```python
from build123d import *

# Parameters (mm, degrees)
SKETCH1_W                 = 131.85
SKETCH1_H                 = 70
BOSS_EXTRUDE1_DEPTH       = 1.5
CUT_EXTRUDE1_REACH        = 137.268
SKETCH4_W                 = 8
SKETCH4_H                 = 4.5
SKETCH4_W_2               = 5
SKETCH4_H_2               = 1.5
BOSS_EXTRUDE2_DEPTH       = 3
MIRROR2_COPY_1_SKETCH_W   = 8
MIRROR2_COPY_1_SKETCH_H   = 4.5
MIRROR2_COPY_1_SKETCH_W_2 = 5
MIRROR2_COPY_1_SKETCH_H_2 = 1.5
MIRROR2_COPY_1_DEPTH      = 3
CUT_EXTRUDE2_REACH        = 137.335
CUT_EXTRUDE3_DEPTH        = 0.5


with BuildPart() as part:
    # Sketch1 → Boss-Extrude1 (new body)
    with BuildSketch(Plane.XY):
        with Locations((55.175, 25.25)):
            Rectangle(SKETCH1_W, SKETCH1_H)
    extrude(amount=BOSS_EXTRUDE1_DEPTH)

    # Sketch2 → Cut-Extrude1 (cut, up to next)
    with BuildSketch(Plane.XY.offset(1.5), mode=Mode.PRIVATE) as cut_extrude1_sk1:
        with BuildLine():
            Line((92.957060126, 22.2), (92.9875, 22.2))
            ThreePointArc((92.9875, 22.2), (96.0375, 25.25), (92.9875, 28.3))
            Line((92.9875, 28.3), (92.957060126, 28.3))
            ThreePointArc((92.957060126, 28.3), (81.0375, 25.25), (92.957060126, 22.2))
        make_face()
    cut_extrude1_tool1 = extrude(cut_extrude1_sk1.sketch, amount=-CUT_EXTRUDE1_REACH, mode=Mode.PRIVATE) & part.part
    add(cut_extrude1_tool1.solids().sort_by_distance((87.98685, 25.25, 1.5))[0], mode=Mode.SUBTRACT)

    # Sketch4 → Boss-Extrude2 (add)
    with BuildSketch(Plane(origin=(0, 0, 0), x_dir=(-1, 0, 0), z_dir=(0, 0, -1))):
        with Locations((-115.6, 56.5)):
            Rectangle(SKETCH4_W, SKETCH4_H)
        with Locations((-115.6, 56.5)):
            Rectangle(SKETCH4_W_2, SKETCH4_H_2, mode=Mode.SUBTRACT)
    boss_extrude2 = extrude(amount=BOSS_EXTRUDE2_DEPTH)

    # Mirror1: Boss-Extrude2 across plane
    add(boss_extrude2.mirror(Plane.ZX.offset(25.25)))

    # Mirror2: Boss-Extrude2 across plane
    add(boss_extrude2.mirror(Plane(origin=(55.175, 0, 0), x_dir=(0, 0, 1), z_dir=(1, 0, 0))))

    # Mirror2 copy 1 sketch → Mirror2 copy 1 (add)
    with BuildSketch(Plane(origin=(110.35, 50.5, 0), x_dir=(1, 0, 0), z_dir=(0, 0, -1))):
        with Locations((-115.6, 56.5)):
            Rectangle(MIRROR2_COPY_1_SKETCH_W, MIRROR2_COPY_1_SKETCH_H)
        with Locations((-115.6, 56.5)):
            Rectangle(MIRROR2_COPY_1_SKETCH_W_2, MIRROR2_COPY_1_SKETCH_H_2, mode=Mode.SUBTRACT)
    extrude(amount=MIRROR2_COPY_1_DEPTH)

    # Sketch5 → Cut-Extrude2 (cut, up to next)
    with BuildSketch(Plane.XY.offset(1.5), mode=Mode.PRIVATE) as cut_extrude2_sk1:
        with BuildLine():
            Line((90.774215328, 6.046350365), (96.908092333, 0.244034279))
            ThreePointArc((96.908092333, 0.244034279), (60.630444856, 25.25), (96.908092333, 50.255965721))
            Line((96.908092333, 50.255965721), (90.774215328, 44.453649635))
            ThreePointArc((90.774215328, 44.453649635), (67.8875, 25.25), (90.774215328, 6.046350365))
        make_face()
    cut_extrude2_tool1 = extrude(cut_extrude2_sk1.sketch, amount=-CUT_EXTRUDE2_REACH, mode=Mode.PRIVATE) & part.part
    add(cut_extrude2_tool1.solids().sort_by_distance((61.276961, 25.25, 1.5))[0], mode=Mode.SUBTRACT)

    # Sketch6 → Cut-Extrude3 (cut)
    with BuildSketch(Plane.XY.offset(1.5)):
        Polygon((-5.119922612, 25.25), (43.3775, -2.75), (43.3775, 6.583333333), (11.045884925, 25.25), (43.3775, 43.916666667), (43.3775, 53.25), align=None)
    extrude(amount=-CUT_EXTRUDE3_DEPTH, mode=Mode.SUBTRACT)


solid = part.part
```
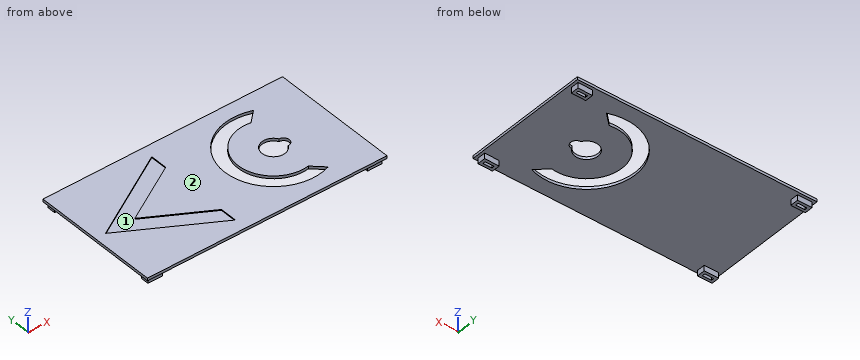
Geometry: final body of the model. Coordinates: model frame, mm. Face numbers are marked on the shaded views. Coordinates: 2 decimals unless noted, no trailing zeros. Order: outer loops, then holes, each group sorted by start corner. A loop starts at its lowest first (then second) coordinate and runs counter-clockwise, first axis right, second up. Notation, with made-up numbers: (69, 64) -> (117, 64) arc R14 ccw to (117, 79) -> close; hole circle Ø11 at (-33.75, 58). An arc over 180 degrees is marked (long way). Write each question's results on one line, items separated by ' | '. Start each with the question number.
1) Material intervals for line 1 along X through (y, z) = (25.25, 0.7); line 2 along X through (y, z) = (56, -0.45); line 3 along Y through (x, z) = (29, 1.25), sorted ascending.
2) First-contact query: pin 1 (2.5 mm diameter, centred on y = 56.5, z = -1.5, fed in from -X); pin 2 (0.9 mm diameter, centred on x = 115.5, z = -2, fed in from -Y); pin 3 (1 mm diameter, centred on x = 45, y = 22, fed in from -Z); pin 4 (2.5 mm diameter, centred on y = -6.5, z = -1, fed in from -X). Flat tips, straight axial feed; report the tip coordinate or a pass-through.
3) Cut plane C-C, the plane x = 105.5. Output: boundary loops of the cut face in (y, z), and give its area (3 significant figures).
4) Cut plane A-A, the plane z = -1.4. State how many separate pieces and enclosed holes the cut face has, and give its area (3 significant figures).
5) Mould query, pull axis Y, two halves, no side actions, for the marked faces 1 and 2. Classes: released by +Y, released by -Y, zero draft, split by the parting line, or undercut.
6) Cut plane B-B, the plane x = 70. Output: boundary loops of the cut face in (y, z), and give its area (3 significant figures).
Checks:
1) line 1: -10.75 to 60.63, 67.89 to 81.04, 96.04 to 121.1 | line 2: -9.25 to -7.75, -2.75 to -1.25, 111.6 to 113.1, 118.1 to 119.6 | line 3: -9.75 to 5.55, 14.88 to 35.62, 44.95 to 60.25
2) pin 1: x = -9.25 | pin 2: y = -8.25 | pin 3: z = 0 | pin 4: x = -10.75
3) outline: (-9.75, 0) -> (60.25, 0) -> (60.25, 1.5) -> (-9.75, 1.5) -> close | area: 105 mm^2
4) separate pieces: 4 | enclosed holes: 4 | area: 114 mm^2
5) face 1: undercut | face 2: zero draft
6) outline: (-9.75, 0) -> (4.91, 0) -> (4.91, 1.5) -> (-9.75, 1.5) -> close; (16.42, 0) -> (34.08, 0) -> (34.08, 1.5) -> (16.42, 1.5) -> close; (45.59, 0) -> (60.25, 0) -> (60.25, 1.5) -> (45.59, 1.5) -> close | area: 70.5 mm^2
